from build123d import *

# Parameters (mm, degrees)
CROQUIS1_W                         = 80
CROQUIS1_H                         = 250
SALIENTE_EXTRUIR1_DEPTH            = 18
CROQUIS2_W                         = 19
CROQUIS2_H                         = 250
CORTAR_EXTRUIR1_DEPTH              = 1
MATRIZL1_COUNT                     = 13
MATRIZL1_PITCH                     = 20
MATRIZL1_COUNT_DIR2                = 2
MATRIZL1_PITCH_DIR2                = 51
TALADROS_DE_ESPIGA_DE_4_0MM1_D     = 4
TALADROS_DE_ESPIGA_DE_4_0MM1_DEPTH = 12
TALADROS_DE_ESPIGA_DE_4_0MM1_TIP   = 1.201721238
TALADRO_ROSCADO_M41_D              = 3.3
TALADRO_ROSCADO_M41_DEPTH          = 11.5
TALADRO_ROSCADO_M41_TIP            = 0.991420021


with BuildPart() as part:
    # Croquis1 → Saliente-Extruir1 (new body)
    with BuildSketch(Plane.XY):
        with Locations((40, 125)):
            Rectangle(CROQUIS1_W, CROQUIS1_H)
    extrude(amount=SALIENTE_EXTRUIR1_DEPTH)

    # Croquis2 → Cortar-Extruir1 (cut)
    with BuildSketch(Plane.XY.offset(18)):
        with Locations((9.5, 125)):
            Rectangle(CROQUIS2_W, CROQUIS2_H)
        with Locations((70.5, 125)):
            Rectangle(CROQUIS2_W, CROQUIS2_H)
    extrude(amount=-CORTAR_EXTRUIR1_DEPTH, mode=Mode.SUBTRACT)

    # Croquis4 → Taladro roscado M31 (revolve, cut)
    with BuildSketch(Plane(origin=(14.5, 245, 17), x_dir=(0, -1, 0), z_dir=(1, 0, 0))):
        Polygon((0, 0), (0, 10.751075774), (1.25, 10), (1.25, 0), align=None)
    taladro_roscado_m31 = revolve(axis=Axis((14.5, 245, 23.35), (0, 0, -1)), mode=Mode.SUBTRACT)

    # MatrizL1: Taladro roscado M31 13 × 2
    with Locations(*[(j * MATRIZL1_PITCH_DIR2, -i * MATRIZL1_PITCH, 0) for i in range(MATRIZL1_COUNT) for j in range(MATRIZL1_COUNT_DIR2) if (i, j) != (0, 0)]):
        add(taladro_roscado_m31, mode=Mode.SUBTRACT)

    # Taladros de espiga de Ø4.0mm1
    with Locations(Plane(origin=(0, 250, 0), x_dir=(1, 0, 0), z_dir=(0, 1, 0))):
        with Locations((60, -9), (20, -9)):
            Hole(TALADROS_DE_ESPIGA_DE_4_0MM1_D / 2, depth=TALADROS_DE_ESPIGA_DE_4_0MM1_DEPTH)
            with Locations((0, 0, -(TALADROS_DE_ESPIGA_DE_4_0MM1_DEPTH + TALADROS_DE_ESPIGA_DE_4_0MM1_TIP / 2))):  # 118° drill point
                Cone(0, TALADROS_DE_ESPIGA_DE_4_0MM1_D / 2, TALADROS_DE_ESPIGA_DE_4_0MM1_TIP, mode=Mode.SUBTRACT)

    # Taladro roscado M41
    with Locations(Plane(origin=(0, 0, 0), x_dir=(-1, 0, 0), z_dir=(0, 0, -1))):
        with Locations((-73.5, 196), (-6.5, 237), (-73.5, 237), (-6.5, 196)):
            Hole(TALADRO_ROSCADO_M41_D / 2, depth=TALADRO_ROSCADO_M41_DEPTH)
            with Locations((0, 0, -(TALADRO_ROSCADO_M41_DEPTH + TALADRO_ROSCADO_M41_TIP / 2))):  # 118° drill point
                Cone(0, TALADRO_ROSCADO_M41_D / 2, TALADRO_ROSCADO_M41_TIP, mode=Mode.SUBTRACT)


solid = part.part
Read the model definition and answer for the solid it produces. Units are mm, in the model's axes. A direction names the side the tool comes from. Coordinates: 2 decimals unless noted, no trailing zeros. Answer in a Markdown table with one row per item.
Item 1: For a pull along Z with two mould halves and no side action, classify faces 1 (the flat face through (40, 127, 18)), 2 (the cylindrical face through (58.092, 243.916, 8.399)), 3 (the flat face through (0, 123, 8)) as released by +Z, released by -Z, zero draft, split by the parting line, or undercut.
Returned:
| item | result |
|---|---|
| face 1 | released by +Z |
| face 2 | undercut |
| face 3 | zero draft |
Item 2: This flat-tipped pin is pushed along its axis until it touches: P1, Ø3, axis at x = 65.5, y = 45, coming from the +Z side. Where does it stop, or does it pass through?
Returned:
| item | result |
|---|---|
| P1 | stops at z = 17 |
Item 3: Straight lines are drawn through the part: line 1 along X through (y, z) = (245, 11.75); line 2 along X through (y, z) = (196, 6); line 3 along Y through (x, z) = (8, 2). For each, find the intervals that lie inside material, in ascending order. Write a range as [from, to].
Returned:
| item | result |
|---|---|
| line 1 | x = [0, 13.25], [15.75, 64.25], [66.75, 80] |
| line 2 | x = [0, 4.85], [8.15, 71.85], [75.15, 80] |
| line 3 | y = [0, 195.31], [196.69, 236.31], [237.69, 250] |
Item 4: For faces 4 (the flat face through (70, 127, 17)), 5 (the flat face through (9, 127, 17)), 6 (the cylindrical face through (21.474, 243.916, 7.648)), 7 (the flat face through (80, 123, 8)), determine the directions among +Z, -Z, +X, -X, +Y, -Y from which every point of the face is accessible in a straight line to the end or side of a thin tool.
Returned:
| item | result |
|---|---|
| face 4 | +Z, +X, +Y, -Y |
| face 5 | +Z, -X, +Y, -Y |
| face 6 | +Y |
| face 7 | +Z, -Z, +X, +Y, -Y |
